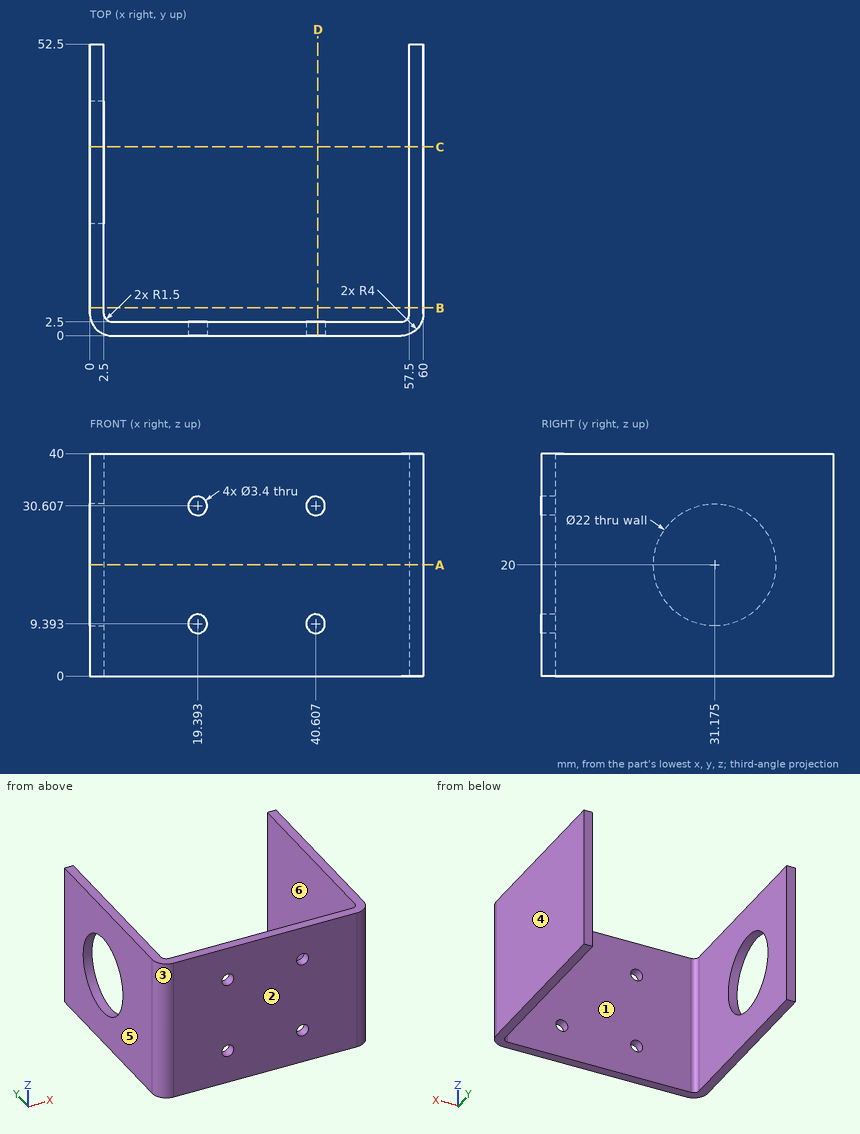
Verification items for this drawing (mm, ordinates from the low corner). A direction names the side the tool comes from. Give positions to 0.01 mm unless a question says otherwise; leave off trailing zeros. Order: outer loops, then holes, each group sorted by start corner. A loop starts at its lowest first (then second) coordinate and runs counter-clockwise, first axis right, second up. Notation, with made-up numbers: M -19,-5 L 33,-5 A15 ccw 33,1 Z; hole C 55,9 d10. An arc over 180 degrees is marked long. Use a Markdown table: item, result.
Item 1: Tool access check on the marked faces 5 and 6. Record the directions out of +Z, -Z, +X, -X, +Y, -Y that give a thin tool (end or side, any length) a straight path to the whole face; none if there is none.
Answers follow:
| item | result |
|---|---|
| face 5 | +Z, -Z, -X, +Y, -Y |
| face 6 | +Z, -Z, +Y |
Item 2: Section check D-D (x = 41). Record the cut outline in (y, z).
Answers follow:
| item | result |
|---|---|
| outline | M 0,0 L 2.5,0 L 2.5,7.74 L 0,7.74 Z; M 0,11.05 L 2.5,11.05 L 2.5,28.95 L 0,28.95 Z; M 0,32.26 L 2.5,32.26 L 2.5,40 L 0,40 Z |
Item 3: Section check B-B (y = 5). Record the cut outline in (x, z).
Answers follow:
| item | result |
|---|---|
| outline | M 0,0 L 2.5,0 L 2.5,40 L 0,40 Z; M 57.5,0 L 60,0 L 60,40 L 57.5,40 Z |
Item 4: Depth check by flat-ended pin: P1, Ø5, axis at x = 11.5, z = 28, coming from the +Y side; P2, Ø8, axis at y = 36, z = 11, coming from the -X side. Enter the tip coordinate at first touch or a pass-through.
Answers follow:
| item | result |
|---|---|
| P1 | stops at y = 2.5 |
| P2 | stops at x = 0 |
Item 5: Material ranges on line 1 along X through (y, z) = (9.5, 19.5); line 2 along Y through (x, z) = (13, 18); line 3 along X through (y, z) = (32, 12), recorded low to high.
Answers follow:
| item | result |
|---|---|
| line 1 | x = 0 to 2.5, 57.5 to 60 |
| line 2 | y = 0 to 2.5 |
| line 3 | x = 57.5 to 60 |
Item 6: Section check C-C (y = 34). Record the cut outline in (x, z).
Answers follow:
| item | result |
|---|---|
| outline | M 0,0 L 2.5,0 L 2.5,9.37 L 0,9.37 Z; M 0,30.63 L 2.5,30.63 L 2.5,40 L 0,40 Z; M 57.5,0 L 60,0 L 60,40 L 57.5,40 Z |
Item 7: Section check A-A (z = 20). Record the cut outline in (x, y) (1 decimal).
Answers follow:
| item | result |
|---|---|
| outline | M 0,4 A4 ccw 4,0 L 56,0 A4 ccw 60,4 L 60,52.5 L 57.5,52.5 L 57.5,4 A1.5 cw 56,2.5 L 4,2.5 A1.5 cw 2.5,4 L 2.5,20.2 L 0,20.2 Z; M 0,42.2 L 2.5,42.2 L 2.5,52.5 L 0,52.5 Z |
Item 8: Draft check along X on the marked faces 1, 2, 3 and 4. Enter one of: +X half, -X half, draft (parallel to the pull), parting line (faces both ways), or undercut.
Answers follow:
| item | result |
|---|---|
| face 1 | undercut |
| face 2 | draft |
| face 3 | -X half |
| face 4 | +X half |
